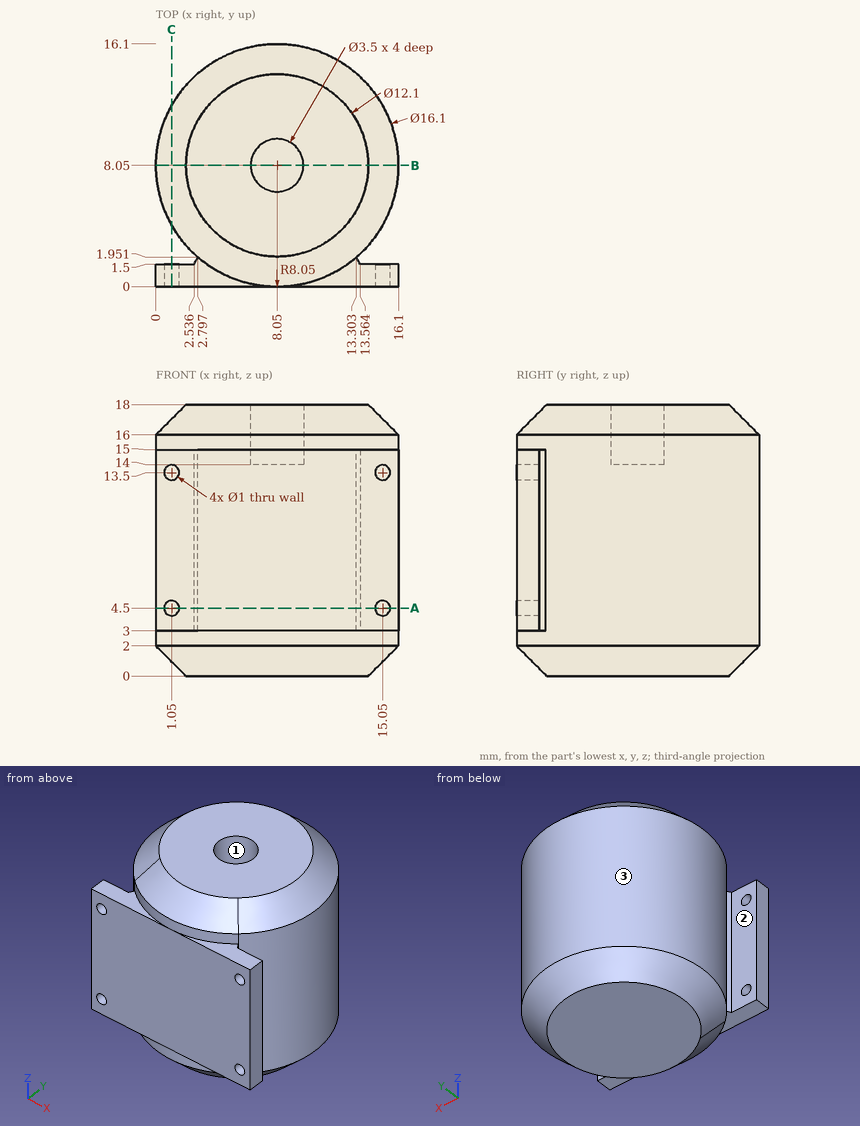
Print and shaded views of the part. All mm, measured from the part's lowest x, y and z. Round coordinates to 2 decimals unless told otherwise and drop trailing zeros. Write each loop counter-clockwise with the first axis right and the second up, starting at its lowest first coordinate (ties: lowest second). Pieces come first, ordered by that corner, then holes. Notation, with made-up numbers: M 57.5,61.25 L 94.5,61.25 A21 ccw 94.5,77.25 Z; hole C 27,-37.5 d6. An arc over 180 degrees is marked long. One line per question, with ' | ' between items.
(1) Probe line 1 along Z through (x, y) = (1.05, 0.4); line 2 along Z through (x, y) = (7.25, 7.75); line 3 along Y through (x, z) = (10.75, 9.75) (1 decimal). List the from-to ranges inside material, lowest first.
Answer key:
line 1: z = 3 to 4, 5 to 13, 14 to 15 | line 2: z = 0 to 14 | line 3: y = 0 to 15.6
(2) Pin check, flat tips, straight feed: pin 1 (0.6 mm diameter, centred on x = 12.5, y = 0.5, fed in from -Z); pin 2 (1 mm diameter, centred on y = 9, z = 5.5, fed in from -X); pin 3 (2 mm diameter, centred on x = 13.5, y = 0.5, fed in from +Z). Stop position of each tip, or through.
Answer key:
pin 1: stops at z = 3 | pin 2: stops at x = 0.01 | pin 3: stops at z = 15
(3) Saw through at B-B on y = 8.05. Write the cut outline in (x, z).
Answer key:
outline: M 0,2 L 2,0 L 14.1,0 L 16.1,2 L 16.1,16 L 14.1,18 L 9.8,18 L 9.8,14 L 6.3,14 L 6.3,18 L 2,18 L 0,16 Z
(4) Saw through at C-C on x = 1.05. Count the separate pieces of the cut face and the enclosed holes in it, then the cut area to 3 significant figures.
Answer key:
separate pieces: 4 | enclosed holes: 0 | area: 137 mm^2
(5) Saw through at A-A on z = 4.5. Write the cut outline in (x, y).
Answer key:
outline: M 0,0 L 0.55,0 L 0.55,1.5 L 0,1.5 Z; M 1.55,0 L 14.55,0 L 14.55,1.5 L 13.56,1.5 L 13.3,1.95 A8.05 ccw long 2.8,1.95 L 2.54,1.5 L 1.55,1.5 Z; M 15.55,0 L 16.1,0 L 16.1,1.5 L 15.55,1.5 Z
(6) Two-plate mould, pull along X, no slides. Class the marked faces 1, 2 and 3: released by +X, released by -X, zero draft, split by the parting line, or undercut.
Answer key:
face 1: undercut | face 2: zero draft | face 3: split by the parting line
